Design review of the part built by this model. Coordinates are the model's own, in mm. A direction names the side the tool comes from. Give positions to 0.01 mm unless a question says otherwise; leave off trailing zeros. Write each loop counter-clockwise with the first axis right and the second up, starting at its lowest first coordinate (ties: lowest second). Pieces come first, ordered by that corner, then holes.
```python
from build123d import *

# Parameters (mm, degrees)
F1_DEPTH = 63.5
F0_W     = 35.0718458849
F0_H     = 19.05
F2_DEPTH = 25.4
F3_DEPTH = 7.9375
F4_W     = 25.4
F4_H     = 19.05
F6_R     = 6.35


with BuildPart() as f1:
    # F0 (on Front) → F1 (new body, symmetric)
    with BuildSketch(Plane.XZ):
        Polygon((41.275, -9.525), (41.275, 9.525), (22.225, 9.525), (-41.275, 9.525), (-41.275, -9.525), align=None)
    extrude(amount=F1_DEPTH, both=True)

    # F0 (on Front) → F2 (join, symmetric)
    with BuildSketch(Plane.XZ):
        with BuildLine():
            Line((22.225, 9.525), (41.275, 9.525))
            Line((41.275, 9.525), (41.275, 27.0002))
            ThreePointArc((41.275, 27.0002), (45.9246798487, 38.2255201513), (57.15, 42.8752))
            Line((57.15, 42.8752), (60.325, 42.8752))
            Line((60.325, 42.8752), (60.325, 61.9252))
            Line((60.325, 61.9252), (57.15, 61.9252))
            ThreePointArc((57.15, 61.9252), (32.4542956671, 51.6959043329), (22.225, 27.0002))
            Line((22.225, 27.0002), (22.225, 9.525))
        make_face()
        with Locations((77.8609229425, 52.4002)):
            Rectangle(F0_W, F0_H)
    extrude(amount=F2_DEPTH, both=True)

    # F0 (on Front) → F3 (join, symmetric)
    with BuildSketch(Plane.XZ):
        with BuildLine():
            Line((-41.275, 9.525), (22.225, 9.525))
            Line((22.225, 9.525), (22.225, 27.0002))
            ThreePointArc((22.225, 27.0002), (32.4542956671, 51.6959043329), (57.15, 61.9252))
            add(Edge.make_bspline(
                [(-41.275, 9.525), (-41.3783525219, 40.9650179304), (3.1078325119, 62.4104812741), (57.15, 61.9252)],
                knots=[0, 0, 0, 0, 111.5045361635, 111.5045361635, 111.5045361635, 111.5045361635], degree=3))
        make_face()
    extrude(amount=F3_DEPTH, both=True)

    # F4 (on face) → F5 (revolve)
    with BuildSketch(Plane.YZ.offset(95.3968458849)):
        with Locations((-12.7, 52.4002)):
            Rectangle(F4_W, F4_H)
    revolve(axis=Axis((95.3968458849, 0, 52.4002), (0, 0, -1)))

    # F6
    f6_edges = [f1.edges().sort_by_distance(p)[0] for p in [
        (41.275, -63.5, 0),
        (41.275, 63.5, 0),
        (-41.275, 63.5, 0),
        (-41.275, -63.5, 0),
    ]]
    fillet(f6_edges, radius=F6_R)


solid = f1.part
```
(1) Consider section C-C, the plane x = 105. Give the boundary of the cut face in (y, z), then the cut area to 3 significant figures.
Resolved:
outline: (-23.51, 42.88) - (23.51, 42.88) - (23.51, 61.93) - (-23.51, 61.93) - close
area: 896 mm2
(2) Consider section A-A, the plane z = 2. Give the boundary of the cut face in (x, y) (3 decimals).
Resolved:
outline: (-41.275, -57.15) arc R6.35 ccw to (-34.925, -63.5) - (34.925, -63.5) arc R6.35 ccw to (41.275, -57.15) - (41.275, 57.15) arc R6.35 ccw to (34.925, 63.5) - (-34.925, 63.5) arc R6.35 ccw to (-41.275, 57.15) - close
(3) Tool access review of faces 1 (the face through (22.225, 17, 18)), 2 (the face through (50, -25.4, 42)), 3 (the face through (22.225, -17, 18)): name each direction out of +Z, -Z, +X, -X, +Y, -Y from which nothing blocks a thin tool from reaching the whole face with its end or side.
Resolved:
face 1: +Z, -X, +Y
face 2: +Z, +X, -X, -Y
face 3: +Z, -X, -Y
(4) Consider section B-B, the plane x = 88. Give the boundary of the cut face in (y, z).
Resolved:
outline: (-25.4, 42.88) - (25.4, 42.88) - (25.4, 61.93) - (-25.4, 61.93) - close
(5) Clearance check with flat-ended pins moving along their axes: P1, Ø6, axis at x = 81.5, y = 12, coming from the -Z side; P2, Ø8, axis at x = 41, z = 28, coming from the +Y side; P3, Ø11, axis at y = 21.5, z = 16.5, coming from the +X side (3 decimals). State where each tip first meets the part, or that it passes through.
Resolved:
P1: stops at z = 42.88
P2: stops at y = 25.4
P3: stops at x = 41.275
(6) To check wall thickness, follow L1, parallel to Y at x = -8, z = 47; L2, parallel to Z at x = 72, y = 11; L3, parallel to Z at x = 33, y = 56 (3 decimals). State the ranges of each line that lie inside material, in increasing order.
Resolved:
L1: y = -7.94 to 7.94
L2: z = 42.88 to 61.93
L3: z = -9.525 to 9.525
